```python
from build123d import *

# Parameters (mm, degrees)
SKETCH1_R           = 2.5
BOSS_EXTRUDE1_DEPTH = 10
SKETCH3_R           = 10
SKETCH3_R_2         = 2.5
BOSS_EXTRUDE2_DEPTH = 2


with BuildPart() as part:
    # Sketch1 → Boss-Extrude1 (new body)
    with BuildSketch(Plane(origin=(0, 0, 0), x_dir=(1, 0, 0), z_dir=(0, 1, 0))):
        Circle(SKETCH1_R)
        with BuildLine():
            Line((-1.242447099, 0.840431559), (0.968768208, 1.14513458))
            ThreePointArc((0.968768208, 1.14513458), (0.204756352, -1.485907091), (-1.242447099, 0.840431559))
        make_face(mode=Mode.SUBTRACT)
    extrude(amount=BOSS_EXTRUDE1_DEPTH)

    # Sketch3 → Boss-Extrude2 (add)
    with BuildSketch(Plane(origin=(0, 10, 0), x_dir=(1, 0, 0), z_dir=(0, 1, 0))):
        Circle(SKETCH3_R)
        Circle(SKETCH3_R_2, mode=Mode.SUBTRACT)
    extrude(amount=-BOSS_EXTRUDE2_DEPTH)


solid = part.part
```
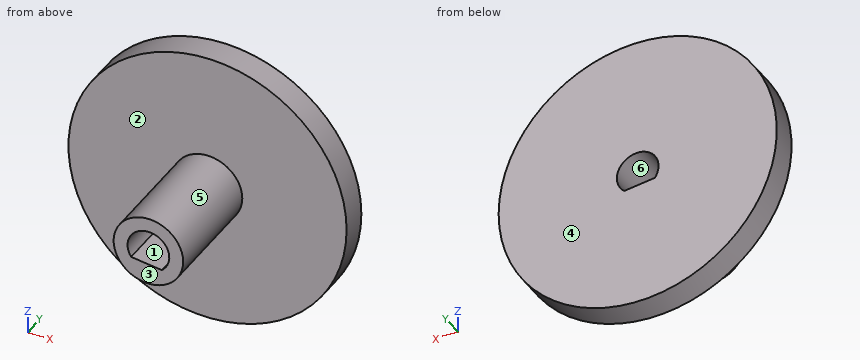
The model under review builds one solid part; all positions refer to its coordinate system, in mm. Face numbers are marked on the shaded views. A direction names the side the tool comes from. Coordinates: 2 decimals unless noted, no trailing zeros. Write each loop counter-clockwise with the first axis right and the second up, starting at its lowest first coordinate (ties: lowest second). Pieces come first, ordered by that corner, then holes.
1) We need section C-C on y = 8.75. State the section outline as (x, z) points, then the cut area to 3 significant figures.
2) Clearance check with flat-ended pins moving along their axes: pin 1 Ø1 at (x, z) = (5.5, -6) entering from -Y; pin 2 Ø1.8 at (x, z) = (0, 0) entering from -Y; pin 3 Ø1.5 at (y, z) = (4, 2) entering from -X; pin 4 Ø1.5 at (x, y) = (-3, 3.5) entering from -Z. State where each tip first meets the part, or that it passes through.
3) Machinability: for the marked faces 1, 2 and 3, which of the approach directions +Z, -Z, +X, -X, +Y, -Y give a long, thin tool a straight path to every point of the face, cutting with its end or side? Answer none if there is none.
4) We need section B-B on x = 0. State the section outline as (y, z) points.
5) We need section D-D on z = -2. State the section outline as (x, y) points.
6) The part is to be moulded in two halves that separate along X. For the marked faces 4, 5 and 6, say which applies: pulls with the +X half, pulls with the -X half, needs draft (parallel to the pull), parting line crosses it, or undercut.
7) To check wall thickness, follow probe 1 along Y at (x, z) = (-7.25, 1); probe 2 along Z at (x, y) = (-1, 0.75); probe 3 along Z at (x, y) = (0.5, 5). State the ranges of each line that lie inside material, in increasing order.
8) We need section A-A on z = 0. State the section outline as (x, y) points.
Answer list:
1. outline: circle Ø20 at (0, 0); hole (-1.24, -0.84) - (0.97, -1.15) arc R1.5 ccw (long way) to start
1. area: 308 mm2
2. pin 1: stops at y = 8
2. pin 2: passes through
2. pin 3: stops at x = -2.17
2. pin 4: stops at z = -1.09
3. face 1: +Y, -Y
3. face 2: -Y
3. face 3: +Z, -Z, +X, -X, -Y
4. outline: (0, -2.5) - (8, -2.5) - (8, -10) - (10, -10) - (10, -1.01) - (0, -1.01) - close; (0, 1.5) - (10, 1.5) - (10, 10) - (8, 10) - (8, 2.5) - (0, 2.5) - close
5. outline: (-9.8, 8) - (-1.5, 8) - (-1.5, 0) - (1.5, 0) - (1.5, 8) - (9.8, 8) - (9.8, 10) - (-9.8, 10) - close
6. face 4: needs draft
6. face 5: parting line crosses it
6. face 6: undercut
7. probe 1: y = 8 to 10
7. probe 2: z = -2.29 to -0.87, 1.12 to 2.29
7. probe 3: z = -2.45 to -1.08, 1.41 to 2.45
8. outline: (-10, 8) - (-2.5, 8) - (-2.5, 0) - (-1.5, 0) - (-1.5, 10) - (-10, 10) - close; (1.5, 0) - (2.5, 0) - (2.5, 8) - (10, 8) - (10, 10) - (1.5, 10) - close
